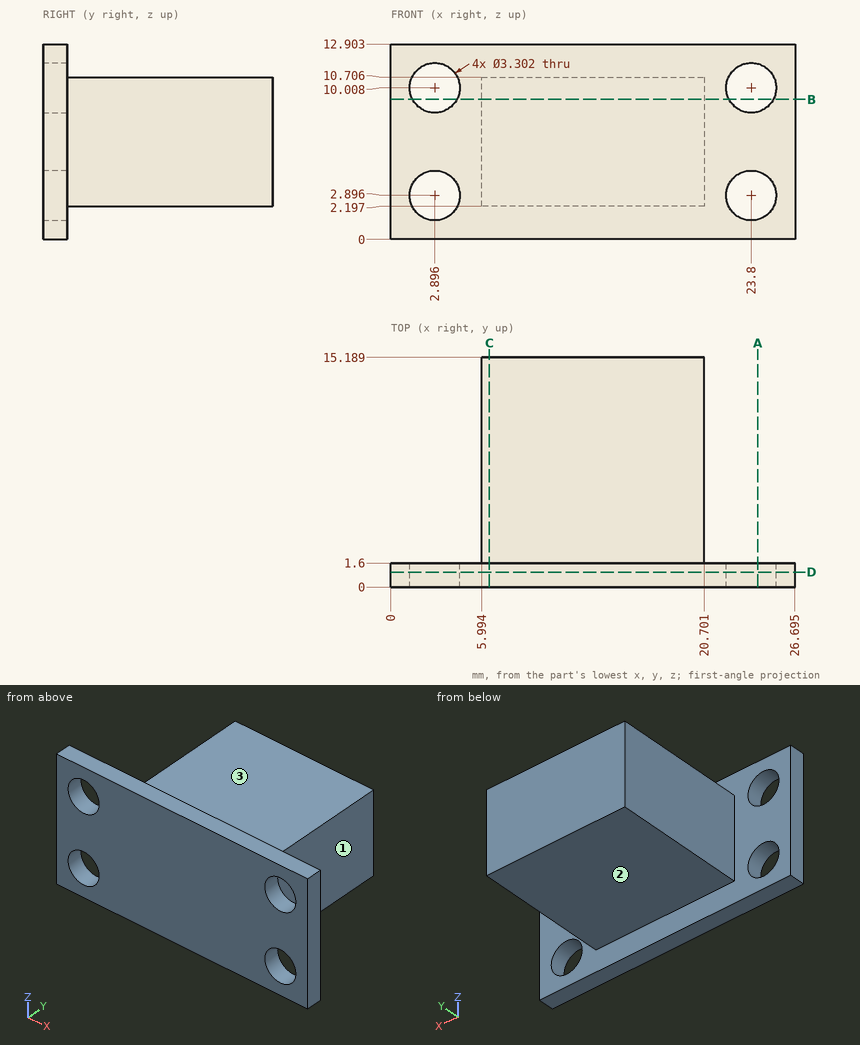
For this review, use the dimensioned drawing (mm, ordinates from the lowest corner) and the shaded views. A direction names the side the tool comes from. Round coordinates to 2 decimals unless told otherwise and drop trailing zeros. Write each loop counter-clockwise with the first axis right and the second up, starting at its lowest first coordinate (ties: lowest second). Pieces come first, ordered by that corner, then holes. Notation, with made-up numbers: (23.25, 12) -> (31.25, 12) arc R25 cw to (31.25, 39) -> close; hole circle Ø5 at (25.25, 15.25). An arc over 180 degrees is marked (long way). Use one line per item in the form item = value.
Q1. Consider section C-C (x = 6.5). State the section outline as (y, z) points.
Resolved:
outline = (0, 0) -> (1.6, 0) -> (1.6, 2.2) -> (15.19, 2.2) -> (15.19, 10.71) -> (1.6, 10.71) -> (1.6, 12.9) -> (0, 12.9) -> close
Q2. Consider section D-D (y = 1). State the section outline as (x, z) points (1 decimal).
Resolved:
outline = (0, 0) -> (26.7, 0) -> (26.7, 12.9) -> (0, 12.9) -> close; hole circle Ø3.3 at (2.9, 2.9); hole circle Ø3.3 at (2.9, 10); hole circle Ø3.3 at (23.8, 2.9); hole circle Ø3.3 at (23.8, 10)
Q3. Consider section B-B (z = 9.25). State the section outline as (x, y) points (1 decimal).
Resolved:
outline = (0, 0) -> (1.4, 0) -> (1.4, 1.6) -> (0, 1.6) -> close; (4.4, 0) -> (22.3, 0) -> (22.3, 1.6) -> (20.7, 1.6) -> (20.7, 15.2) -> (6, 15.2) -> (6, 1.6) -> (4.4, 1.6) -> close; (25.3, 0) -> (26.7, 0) -> (26.7, 1.6) -> (25.3, 1.6) -> close
Q4. Machinability: for the marked faces 1, 2 and 3, which of the approach directions +Z, -Z, +X, -X, +Y, -Y give a long, thin tool a straight path to every point of the face, cutting with its end or side? Answer none if there is none.
Resolved:
face_1 = +Z, -Z, +X, +Y
face_2 = -Z, +X, -X, +Y
face_3 = +Z, +X, -X, +Y
Q5. To check wall thickness, follow probe 1 along X at (y, z) = (10, 8.75) (1 decimal); probe 2 along Z at (x, y) = (12.5, 2.5); probe 3 along Y at (x, z) = (2, 8.25). State the ranges of each line that lie inside material, in increasing order. Write a range as from..to.
Resolved:
probe_1 = 6..20.7
probe_2 = 2.2..10.71
probe_3 = 0..1.6
Q6. Clearance check with flat-ended pins moving along their axes: pin 1 Ø7 at (x, y) = (9.5, 10) entering from -Z; pin 2 Ø2 at (y, z) = (9.5, 4.5) entering from +X; pin 3 Ø6 at (x, y) = (7.5, 13.5) entering from +Z. State where each tip first meets the part, or that it passes through.
Resolved:
pin_1 = 2.2
pin_2 = 20.7
pin_3 = 10.71
Q7. Consider section A-A (x = 24.25). State the section outline as (y, z) points, then the cut area to 3 significant figures.
Resolved:
outline = (0, 0) -> (1.6, 0) -> (1.6, 1.31) -> (0, 1.31) -> close; (0, 4.48) -> (1.6, 4.48) -> (1.6, 8.42) -> (0, 8.42) -> close; (0, 11.6) -> (1.6, 11.6) -> (1.6, 12.9) -> (0, 12.9) -> close
area = 10.5 mm²
